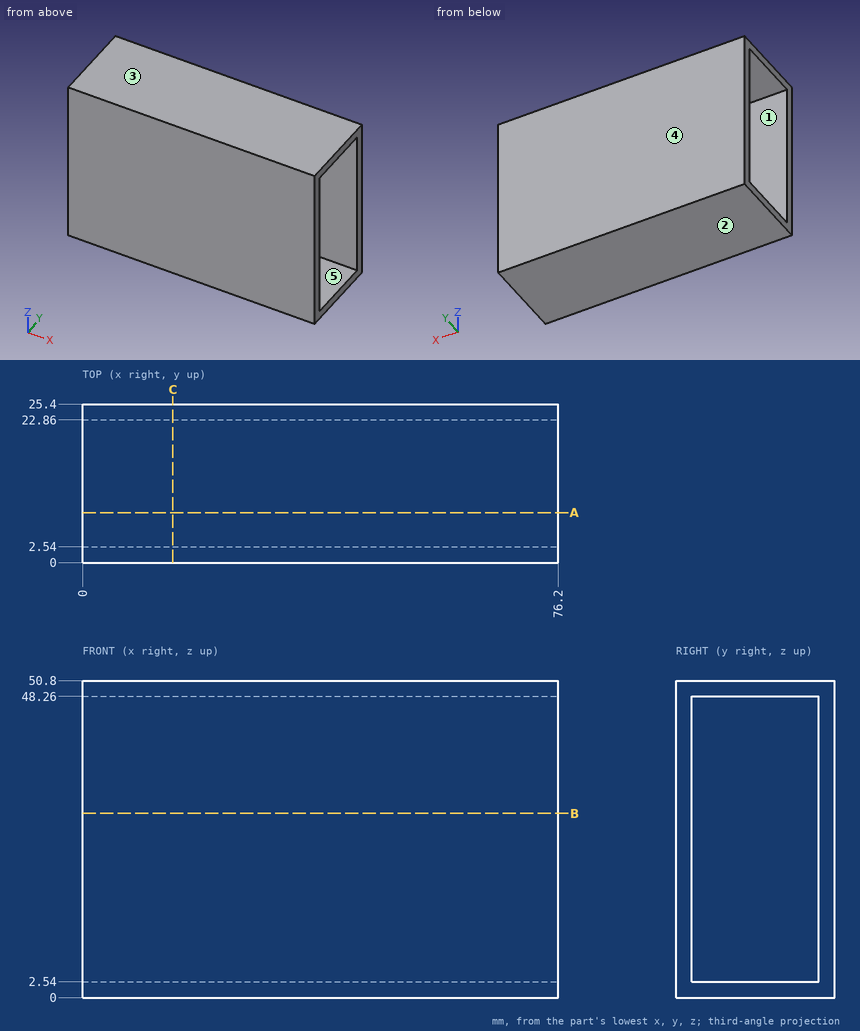
Job drawing, mm, ordinate dimensions from the low corner. One solid piece. A direction names the side the tool comes from. Give positions to 0.01 mm unless a question says otherwise; leave off trailing zeros. Write each loop counter-clockwise with the first axis right and the second up, starting at its lowest first coordinate (ties: lowest second). Pieces come first, ordered by that corner, then holes. Notation, with made-up numbers: M 12,79.25 L 48,79.25 A5 cw 48,86.25 Z; hole C -28.5,-30.75 d4. An arc over 180 degrees is marked long. Put each result on its own line as item: value. Start each with the question number.
(1) Band-saw the part on B-B, the plane z = 29.5. Write the cut outline in (x, y), and give its area (3 significant figures).
(2) Probe L1, parallel to Z at x = 36, y = 6.5; L2, parallel to Y at x = 44, z = 5. List the from-to ranges inside material, lowest first.
(3) Mould opens along Z. For the marked faces 1, 2 and 3 say: +Z half, -Z half, draft (parallel to the pull), parting line (faces both ways), or undercut.
(4) Flat gauge pins, fed straight in: pin 1 Ø12 at (y, z) = (22, 24.5) entering from -X; pin 2 Ø12 at (y, z) = (9.5, 10.5) entering from +X. Where does each tip first touch, or does it go through?
(5) Band-saw the part on A-A, the plane y = 8. Write the cut outline in (x, z).
(6) Band-saw the part on C-C, the plane x = 14.5. Write the cut outline in (y, z), and give its area (3 significant figures).
(7) Which spindle directions (+Z, -Z, +X, -X, +Y, -Y) get a long thin tool onto all of the face, cutting with end or side? Do the marked faces 4 and 5. Say none if no direction does.
Response values:
1. outline: M 0,0 L 76.2,0 L 76.2,2.54 L 0,2.54 Z; M 0,22.86 L 76.2,22.86 L 76.2,25.4 L 0,25.4 Z
1. area: 387 mm2
2. L1: z = 0 to 2.54, 48.26 to 50.8
2. L2: y = 0 to 2.54, 22.86 to 25.4
3. face 1: undercut
3. face 2: -Z half
3. face 3: +Z half
4. pin 1: stops at x = 0
4. pin 2: passes through
5. outline: M 0,0 L 76.2,0 L 76.2,2.54 L 0,2.54 Z; M 0,48.26 L 76.2,48.26 L 76.2,50.8 L 0,50.8 Z
6. outline: M 0,0 L 25.4,0 L 25.4,50.8 L 0,50.8 Z; hole M 2.54,2.54 L 22.86,2.54 L 22.86,48.26 L 2.54,48.26 Z
6. area: 361 mm2
7. face 4: +Z, -Z, +X, -X, +Y
7. face 5: +X, -X
